Work out the finished part from the listing and answer in its coordinate system (mm). A direction names the side the tool comes from. Round coordinates to 2 decimals unless told otherwise and drop trailing zeros. Write each loop counter-clockwise with the first axis right and the second up, starting at its lowest first coordinate (ties: lowest second). Pieces come first, ordered by that corner, then holes. Notation, with made-up numbers: (-18.5, 14.5) -> (-8.5, 14.5) arc R21 ccw to (-8.5, 39.5) -> close; hole circle Ø4 at (26.25, -16.75). An arc over 180 degrees is marked (long way). One line per item, written item: value.
```python
from build123d import *

# Parameters (mm, degrees)
SKETCH_1_W               = 28
SKETCH_1_H               = 28
EXTRUDE_1_DEPTH          = 10
SKETCH_2_R               = 9.5
CUT_EXTRUDE_1_DEPTH      = 11
SKETCH_3_R               = 10.55
CUT_EXTRUDE_2_DEPTH      = 8
SKETCH_4_R               = 12.05
CUT_EXTRUDE_3_DEPTH      = 6
FILLET_1_R               = 2
SKETCH_5_R               = 1.3
CUT_EXTRUDE_4_DEPTH      = 11
SKETCH_6_W               = 1
SKETCH_6_H               = 2
EXTRUDE_2_DEPTH          = 3
PATTERN_CIRCULAR_1_COUNT = 4


with BuildPart() as part:
    # 草图1 → 凸台-拉伸1 (new body)
    with BuildSketch(Plane.XY):
        Rectangle(SKETCH_1_W, SKETCH_1_H)
    extrude(amount=EXTRUDE_1_DEPTH)

    # 草图2 → 切除-拉伸1 (cut, through all)
    with BuildSketch(Plane.XY.offset(10)):
        Circle(SKETCH_2_R)
    extrude(amount=-CUT_EXTRUDE_1_DEPTH, mode=Mode.SUBTRACT)

    # 草图3 → 切除-拉伸2 (cut)
    with BuildSketch(Plane.XY.offset(10)):
        Circle(SKETCH_3_R)
    extrude(amount=-CUT_EXTRUDE_2_DEPTH, mode=Mode.SUBTRACT)

    # 草图4 → 切除-拉伸3 (cut)
    with BuildSketch(Plane.XY.offset(10)):
        Circle(SKETCH_4_R)
    extrude(amount=-CUT_EXTRUDE_3_DEPTH, mode=Mode.SUBTRACT)

    # 圆角1
    fillet_1_edges = [part.edges().sort_by_distance(p)[0] for p in [
        (14, -14, 5),
        (-14, -14, 5),
        (-14, 14, 5),
        (14, 14, 5),
    ]]
    fillet(fillet_1_edges, radius=FILLET_1_R)

    # 草图5 → 切除-拉伸4 (cut, through all)
    with BuildSketch(Plane.XY.offset(10)):
        with Locations((-11.6, 11.6)):
            Circle(SKETCH_5_R)
        with Locations((11.6, 11.6)):
            Circle(SKETCH_5_R)
        with Locations((11.6, -11.6)):
            Circle(SKETCH_5_R)
        with Locations((-11.6, -11.6)):
            Circle(SKETCH_5_R)
    extrude(amount=-CUT_EXTRUDE_4_DEPTH, mode=Mode.SUBTRACT)

    # 草图6 → 凸台-拉伸2 (add)
    with BuildSketch(Plane.XY.offset(10)):
        with Locations((-13.5, -8)):
            Rectangle(SKETCH_6_W, SKETCH_6_H)
    extrude_2 = extrude(amount=EXTRUDE_2_DEPTH)

    # 阵列(圆周)1: 凸台-拉伸2 ×4 about axis
    pattern_circular_1_axis = Axis((0, 0, 0), (0, 0, 1))
    for i in range(1, PATTERN_CIRCULAR_1_COUNT):
        add(extrude_2.rotate(pattern_circular_1_axis, i * 360 / PATTERN_CIRCULAR_1_COUNT))


solid = part.part
```
(1) A tool of negligible diameter and unlimited length cuts with its end or side. For faces 4 (the face through (13.5, 9, 11.5)), 5 (the face through (0, -11, 4)), 6 (the face through (-7, 13.5, 11.5)), from which of +Z, -Z, +X, -X, +Y, -Y can it reach the whole face along a straight path? Write none if from no direction.
Reported:
face 4: +Z, +X, -X, +Y
face 5: +Z
face 6: +Z, +X, +Y, -Y
(2) Find section D-D on z = 11.5. Give the vertices of the cut face in (x, y), plus the area to 3 significant figures.
Reported:
outline: (-14, -9) -> (-13, -9) -> (-13, -7) -> (-14, -7) -> close; (-9, 13) -> (-7, 13) -> (-7, 14) -> (-9, 14) -> close; (7, -14) -> (9, -14) -> (9, -13) -> (7, -13) -> close; (13, 7) -> (14, 7) -> (14, 9) -> (13, 9) -> close
area: 8.00 mm2
(3) Find section A-A on z = 5.5. Give the vertices of the cut face in (x, y), plus the area to 3 significant figures.
Reported:
outline: (-14, -12) arc R2 ccw to (-12, -14) -> (12, -14) arc R2 ccw to (14, -12) -> (14, 12) arc R2 ccw to (12, 14) -> (-12, 14) arc R2 ccw to (-14, 12) -> close; hole circle Ø2.6 at (-11.6, -11.6); hole circle Ø2.6 at (-11.6, 11.6); hole circle Ø24.1 at (0, 0); hole circle Ø2.6 at (11.6, -11.6); hole circle Ø2.6 at (11.6, 11.6)
area: 303 mm2
(4) Flat-ended cylindrical pins translate along their axes: pin 1 Ø3.5 at (x, y) = (-11.6, -11.6) entering from -Z; pin 2 Ø0.8 at (y, z) = (-13.5, 12) entering from +X; pin 3 Ø0.6 at (y, z) = (7.5, 12) entering from -X; pin 4 Ø1.6 at (x, y) = (11.6, -11.6) entering from -Z. Find the tip coordinate at first contact, or state that the pin passes through.
Reported:
pin 1: stops at z = 0
pin 2: stops at x = 9
pin 3: stops at x = 13
pin 4: passes through
(5) For a pull along Y with two mould halves and no side action, classify faces 1 (the face through (-9, 4, 2)), 2 (the face through (-13, 0, 10)), 3 (the face through (-13.43, -13.4, 5.07)) as pulls with the +Y half, pulls with the -Y half, needs draft (parallel to the pull), parting line crosses it, or undercut.
Reported:
face 1: undercut
face 2: needs draft
face 3: pulls with the -Y half
(6) Consider probe 1 along Y at (x, z) = (0, 1.5); probe 2 along Y at (x, z) = (0, 5.9); probe 3 along Z at (x, y) = (11.5, 6.5). Determine where each line is inside the solid, lowest interval first.
Reported:
probe 1: y = -14 to -9.5, 9.5 to 14
probe 2: y = -14 to -12.05, 12.05 to 14
probe 3: z = 0 to 10
(7) Find section B-B on x = 0. Give the vertices of the cut face in (y, z), plus the area to 3 significant figures.
Reported:
outline: (-14, 0) -> (-9.5, 0) -> (-9.5, 2) -> (-10.55, 2) -> (-10.55, 4) -> (-12.05, 4) -> (-12.05, 10) -> (-14, 10) -> close; (9.5, 0) -> (14, 0) -> (14, 10) -> (12.05, 10) -> (12.05, 4) -> (10.55, 4) -> (10.55, 2) -> (9.5, 2) -> close
area: 55.2 mm2
